from build123d import *

# Parameters (mm, degrees)
SKETCH1_W           = 25.4
SKETCH1_H           = 25.4
BOSS_EXTRUDE1_DEPTH = 3.175
SKETCH2_W           = 6.35
SKETCH2_H           = 3.175
BOSS_EXTRUDE2_DEPTH = 3.175
CUT_EXTRUDE1_DEPTH  = 6.35


with BuildPart() as part:
    # Sketch1 → Boss-Extrude1 (new body)
    with BuildSketch(Plane(origin=(0, 0, 0), x_dir=(1, 0, 0), z_dir=(0, 1, 0))):
        Rectangle(SKETCH1_W, SKETCH1_H)
        Polygon((-4.1275, -4.1275), (-4.1275, 3.95986), (-2.54, 3.95986), (-2.54, -2.54), (3.95986, -2.54), (3.95986, -4.1275), align=None, mode=Mode.SUBTRACT)
    extrude(amount=BOSS_EXTRUDE1_DEPTH)

    # Sketch2 → Boss-Extrude2 (add)
    with BuildSketch(Plane.XY.offset(12.7)):
        with Locations((-9.525, 1.5875)):
            Rectangle(SKETCH2_W, SKETCH2_H)
        with Locations((9.525, 1.5875)):
            Rectangle(SKETCH2_W, SKETCH2_H)
    extrude(amount=BOSS_EXTRUDE2_DEPTH)

    # Sketch3 → Cut-Extrude1 (cut)
    with BuildSketch(Plane(origin=(0, 3.175, 0), x_dir=(1, 0, 0), z_dir=(0, 1, 0))):
        Polygon((-2.54, 2.37236), (-2.54, -2.54), (2.37236, -2.54), align=None)
    extrude(amount=-CUT_EXTRUDE1_DEPTH, mode=Mode.SUBTRACT)


solid = part.part
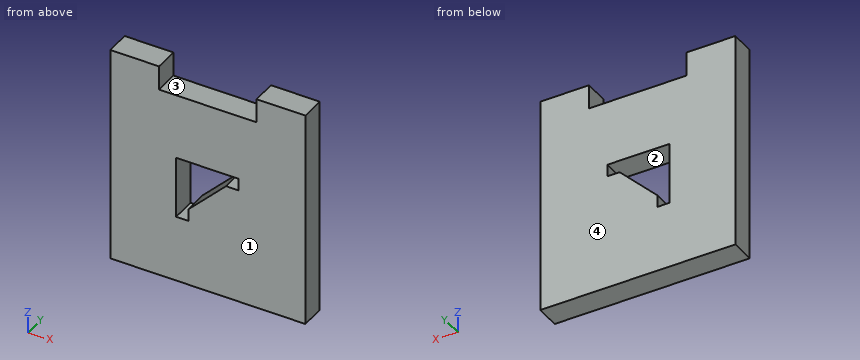
Could you check a few things on this model? Use its own coordinates, in mm. Face numbers are marked on the shaded views. A direction names the side the tool comes from. Give positions to 0.01 mm unless a question says otherwise; leave off trailing zeros. Write each loop counter-clockwise with the first axis right and the second up, starting at its lowest first coordinate (ties: lowest second). Pieces come first, ordered by that corner, then holes. Notation, with made-up numbers: (11, -37.75) -> (22, -37.75) arc R23 ccw to (22, -9.75) -> close; hole circle Ø6 at (-38, 62). An arc over 180 degrees is marked (long way). Write each question's results on one line, items separated by ' | '. Start each with the question number.
Q1. I'm going to push a flat-ended pin straight in: pin 1 Ø1.7 at (x, y) = (3, 1.5) entering from +Z. Where does the tip first touch, or does it pass through?
Q2. Suppose I cut it at C-C, the plane z = -2. List the corners of the cut face in (x, y) for me (1 decimal), and give its area (3 significant figures).
Q3. Which directions (+Z, -Z, +X, -X, +Y, -Y) give clear straight access to the entire face, cutting with the end or side of a thin tool? Please do the marked faces 1 and 2.
Q4. I need wall thicknesses on probe 1 along Z at (x, y) = (-3, 2.55); probe 2 along X at (y, z) = (0.1, 4); probe 3 along Z at (x, y) = (-5.75, 1.7). Which ranges of each line are inside material? Lowest first, please.
Q5. Suppose I cut it at A-A, the plane x = -3. List the corners of the cut face in (y, z) for me (1 decimal), and give its area (3 significant figures).
Q6. Suppose I cut it at D-D, the plane x = -5.75. List the corners of the cut face in (y, z) for me (3 decimals).
Q7. We'd pull the mould along X, two halves only. Please class the marked faces 3 and 4: +X half, -X half, draft (parallel to the pull), parting line (faces both ways), or undercut.
Outcome:
1) pin 1: z = 12.7
2) outline: (-12.7, 0) -> (-4.1, 0) -> (-4.1, 3.2) -> (-12.7, 3.2) -> close; (-2.2, 0) -> (12.7, 0) -> (12.7, 3.2) -> (-2.2, 3.2) -> close | area: 74.4 mm2
3) face 1: +Z, -Z, +X, -X, -Y | face 2: +Y, -Y
4) probe 1: -12.7 to -3.96, 4.13 to 12.7 | probe 2: -12.7 to -4.13, 3.96 to 12.7 | probe 3: -12.7 to 12.7
5) outline: (0, -12.7) -> (3.2, -12.7) -> (3.2, -4) -> (0, -4) -> close; (0, 4.1) -> (3.2, 4.1) -> (3.2, 12.7) -> (0, 12.7) -> close | area: 55.0 mm2
6) outline: (0, -12.7) -> (3.175, -12.7) -> (3.175, 12.7) -> (0, 12.7) -> close
7) face 3: undercut | face 4: draft
